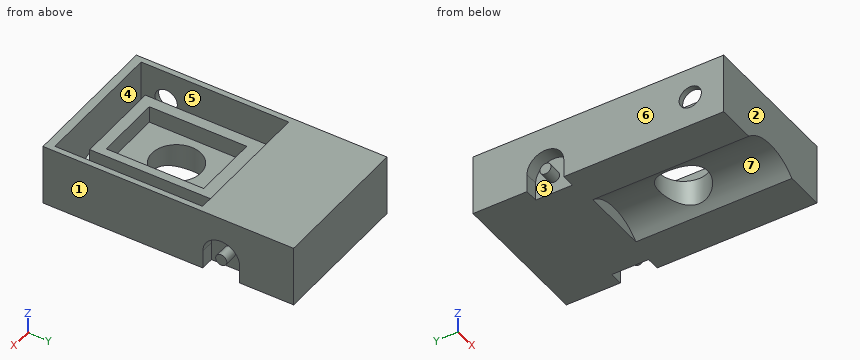
```python
from build123d import *

# Parameters (mm, degrees)
SKETCH1_W           = 26
SKETCH1_H           = 45
BOSS_EXTRUDE1_DEPTH = 11
SKETCH2_R           = 8.45
CUT_EXTRUDE1_DEPTH  = 28
CUT_EXTRUDE2_DEPTH  = 26.5
BOSS_EXTRUDE2_START = 23
BOSS_EXTRUDE2_DEPTH = 23
SKETCH6_W           = 12
SKETCH6_H           = 17.5
CUT_EXTRUDE3_DEPTH  = 3
SKETCH7_R           = 4.4
CUT_EXTRUDE4_DEPTH  = 53.316345438
SKETCH8_R           = 2
CUT_EXTRUDE5_DEPTH  = 3
SKETCH9_R           = 1
CUT_EXTRUDE6_DEPTH  = 2.4
CUT_EXTRUDE7_START  = -2.4
SKETCH10_R          = 1
CUT_EXTRUDE7_DEPTH  = 2.4


with BuildPart() as part:
    # Sketch1 → Boss-Extrude1 (new body)
    with BuildSketch(Plane.XY):
        with Locations((13, -22.5)):
            Rectangle(SKETCH1_W, SKETCH1_H)
    extrude(amount=BOSS_EXTRUDE1_DEPTH)

    # Sketch2 → Cut-Extrude1 (cut)
    with BuildSketch(Plane.XZ.offset(45)):
        with Locations((13, -5.95)):
            Circle(SKETCH2_R)
    extrude(amount=-CUT_EXTRUDE1_DEPTH, mode=Mode.SUBTRACT)

    # Sketch4 → Cut-Extrude2 (cut)
    with BuildSketch(Plane(origin=(0, -43.5, 0), x_dir=(-1, 0, 0), z_dir=(0, -1, 0))):
        with BuildLine():
            Line((-1, -11), (-1, -1))
            Line((-1, -1), (-6.596875763, -1))
            ThreePointArc((-6.596875763, -1), (-13, -3.5), (-19.403124237, -1))
            Line((-19.403124237, -1), (-25, -1))
            Line((-25, -1), (-25, -11))
            Line((-25, -11), (-1, -11))
        make_face()
    extrude(amount=-CUT_EXTRUDE2_DEPTH, mode=Mode.SUBTRACT)

    # Sketch5 → Boss-Extrude2 (add)
    with BuildSketch(Plane.XZ.offset(17).offset(BOSS_EXTRUDE2_START)):
        with BuildLine():
            Line((6.596875763, 1), (5.25, 1))
            Line((5.25, 1), (5.25, 9))
            Line((5.25, 9), (20.75, 9))
            Line((20.75, 9), (20.75, 1))
            Line((20.75, 1), (19.403124237, 1))
            ThreePointArc((19.403124237, 1), (13, 3.5), (6.596875763, 1))
        make_face()
    extrude(amount=-BOSS_EXTRUDE2_DEPTH)

    # Sketch6 → Cut-Extrude3 (cut)
    with BuildSketch(Plane.XY.offset(9)):
        with Locations((13.25, -29.25)):
            Rectangle(SKETCH6_W, SKETCH6_H)
    extrude(amount=-CUT_EXTRUDE3_DEPTH, mode=Mode.SUBTRACT)

    # Sketch7 → Cut-Extrude4 (cut, through all)
    with BuildSketch(Plane.XY.offset(6)):
        with Locations((13.25, -29.25)):
            Circle(SKETCH7_R)
    extrude(amount=-CUT_EXTRUDE4_DEPTH, mode=Mode.SUBTRACT)

    # Sketch8 → Cut-Extrude5 (cut)
    with BuildSketch(Plane.ZY):
        with Locations(Location((5.5, -39, 0), (0, 0, 270))):
            Circle(SKETCH8_R)
    extrude(amount=-CUT_EXTRUDE5_DEPTH, mode=Mode.SUBTRACT)

    # Sketch9 → Cut-Extrude6 (cut)
    with BuildSketch(Plane.ZY):
        with BuildLine():
            Line((0, -16.3), (3.3, -16.3))
            ThreePointArc((3.3, -16.3), (6.6, -13), (3.3, -9.7))
            Line((3.3, -9.7), (0, -9.7))
            Line((0, -9.7), (0, -16.3))
        make_face()
        with Locations(Location((3, -13, 0), (0, 0, 270))):
            Circle(SKETCH9_R, mode=Mode.SUBTRACT)
    extrude(amount=-CUT_EXTRUDE6_DEPTH, mode=Mode.SUBTRACT)

    # Sketch10 → Cut-Extrude7 (cut)
    with BuildSketch(Plane(origin=(26, 0, 0), x_dir=(0, 0, -1), z_dir=(1, 0, 0)).offset(CUT_EXTRUDE7_START)):
        with BuildLine():
            Line((0, -16.3), (0, -9.7))
            Line((0, -9.7), (-3.3, -9.7))
            ThreePointArc((-3.3, -9.7), (-6.6, -13), (-3.3, -16.3))
            Line((-3.3, -16.3), (0, -16.3))
        make_face()
        with Locations(Location((-3, -13, 0), (0, 0, 270))):
            Circle(SKETCH10_R, mode=Mode.SUBTRACT)
    extrude(amount=CUT_EXTRUDE7_DEPTH, mode=Mode.SUBTRACT)


solid = part.part
```
Part model, mm, in its own coordinate system. Face numbers are marked on the shaded views. A direction names the side the tool comes from. Round coordinates to 2 decimals unless told otherwise and drop trailing zeros. Write each loop counter-clockwise with the first axis right and the second up, starting at its lowest first coordinate (ties: lowest second). Pieces come first, ordered by that corner, then holes. Notation, with made-up numbers: M -30.5,39 L -11.5,39 A34 cw -11.5,70 Z; hole C 79.5,64.25 d1. An arc over 180 degrees is marked long. One line per question, with ' | ' between items.
(1) Saw through at D-D on y = -13. Write the cut outline in (x, z).
Answer key:
outline: M 0,2 L 2.4,2 L 2.4,0 L 23.6,0 L 23.6,2 L 26,2 L 26,4 L 23.6,4 L 23.6,6.6 L 26,6.6 L 26,11 L 0,11 L 0,6.6 L 2.4,6.6 L 2.4,4 L 0,4 Z
(2) Saw through at C-C on z = 10. Write the cut outline in (x, y).
Answer key:
outline: M 0,-45 L 26,-45 L 26,0 L 0,0 Z; hole M 1,-43.5 L 25,-43.5 L 25,-17 L 1,-17 Z
(3) Probe line 1 along Y through (x, z) = (13, 4.75); line 2 along X through (y, z) = (-29.25, 2.85); line 3 along X through (y, z) = (-19, 8). List the from-to ranges inside material, lowest first.
Answer key:
line 1: y = -45 to -43.5, -40 to -33.64, -24.86 to 0 | line 2: x = 0 to 1, 5.25 to 8.85, 17.65 to 20.75, 25 to 26 | line 3: x = 0 to 1, 5.25 to 20.75, 25 to 26
(4) Saw through at B-B on y = -39. Write the cut outline in (x, z).
Answer key:
outline: M 0,0 L 7,0 A8.45 cw 19,0 L 26,0 L 26,11 L 25,11 L 25,1 L 20.75,1 L 20.75,9 L 5.25,9 L 5.25,1 L 1,1 L 1,3.5 L 0,3.5 Z; M 0,7.5 L 1,7.5 L 1,11 L 0,11 Z
(5) Saw through at A-A on x = 21.75. Write the cut outline in (y, z), then the cut area to 3 significant figures.
Answer key:
outline: M -45,0 L 0,0 L 0,11 L -17,11 L -17,1 L -43.5,1 L -43.5,11 L -45,11 Z | area: 230 mm^2
(6) Pin check, flat tips, straight feed: pin 1 (3 mm diameter, centred on x = 3, y = -24.5, fed in from +Z); pin 2 (1.2 mm diameter, centred on x = 1, z = 1, fed in from +Y); pin 3 (4 mm diameter, centred on x = 20.5, y = -28, fed in from +Z); pin 4 (2 mm diameter, centred on x = 9, y = -31, fed in from +Z). Stop position of each tip, or through.
Answer key:
pin 1: stops at z = 1 | pin 2: stops at y = 0 | pin 3: stops at z = 9 | pin 4: stops at z = 6
(7) 3-axis set-ups, long thin cutter, end or side, ignore diameter. For the marked faces 5, 6 and 7: which of +Z, -Z, +X, -X, +Y, -Y reach the whole face in a straight line?
Answer key:
face 5: +Z | face 6: +Z, -Z, -X, +Y, -Y | face 7: -Z, -Y
(8) Two-plate mould, pull along X, no slides. Class the marked faces 1, 2, 3 and 4: released by +X, released by -X, zero draft, split by the parting line, or undercut.
Answer key:
face 1: released by +X | face 2: zero draft | face 3: released by -X | face 4: undercut
